Autodesk Inventor part; units mm, degrees
ref_plane "YZ Plane" through (0, 0, 0) normal (1, 0, 0) x (0, 1, 0)
ref_plane "XZ Plane" through (0, 0, 0) normal (0, 1, 0) x (-1, 0, 0)
ref_plane "XY Plane" through (0, 0, 0) normal (0, 0, 1) x (1, 0, 0)
sketch "Skizze1" plane through (0, 0, 0) normal (0, 0, 1) x (1, 0, 0)
  line L0 (0, 0) -> (50, 0)
  line L1 (50, 0) -> (50, 5)
  line L2 (36.2626, 10) -> (0, 10)
  line L3 (0, 10) -> (0, 0)
  line L4 (36.2626, 10) -> (50, 5)
  dimension "d0" = 10
  dimension "d1" = 50
  dimension "d2" = 5
  dimension "d5" = 20
extrude "Extrusion1" add sketch "Skizze1" along normal blind 2
sketch "Skizze2" plane through (0, 0, 2) normal (0, 0, 1) x (1, 0, 0)
  line L0 (0, 0) -> (0, 10)
  line L1 (0, 10) -> (36.2626, 10)
  line L2 (0, 5) -> (28.2614, 5)
  point P0 (4, 5)
  point P1 (12, 5)
  dimension "d8" = 4
  dimension "d9" = 8
hole "Bohrung1" at (4, 5, 2) at (12, 5, 2) direction (0, 0, -1) diameter 3.4 end through all
sketch "Skizze4" plane through (0, 0, 2) normal (0, 0, 1) x (1, 0, 0)
  circle A0 centre (4, 5) radius 1.7
  line L0 (50, 0) -> (0, 0)
  line L1 (0, 10) -> (36.2626, 10)
  line L2 (5.7, 7) -> (5.7, 3)
  line L3 (2.3, 3) -> (2.3, 7)
  arc A1 (5.7, 7) -> (2.3, 7) centre (4, 7) ccw
  arc A2 (2.3, 3) -> (5.7, 3) centre (4, 3) ccw
  dimension "d17" = 3
  dimension "d18" = 3
  dimension "d19" = 4
extrude "Extrusion2" cut sketch "Skizze4" against normal through all contours L2 A2 L3 A0 | A0 L3 A1 L2
pattern_linear "Rechteckige Anordnung1" count 2 spacing 8 along (1, 0, 0) of "Extrusion2"
properties part number "13_0204_068"
Design review of the part built by this model. Coordinates are the model's own, in mm. A direction names the side the tool comes from. Coordinates: 2 decimals unless noted, no trailing zeros. Write each loop counter-clockwise with the first axis right and the second up, starting at its lowest first coordinate (ties: lowest second). Pieces come first, ordered by that corner, then holes. Notation, with made-up numbers: (68, -13.5) - (113, -13.5) arc R8 ccw to (113, 1.5) - close; hole circle Ø6 at (-4, -22). An arc over 180 degrees is marked (long way). Use one line per item in the form item = value.
Q1. Insertion check: pin 1 Ø0.6 at (y, z) = (5.5, 1) entering from -X. The pin has a flat end and moves straight along its axis. Give the tip position at first contact, or say it passes through.
Taken from the geometry:
pin_1 = 0
Q2. Consider section C-C (z = 1.1). Write out the cut boundary in (x, y).
Taken from the geometry:
outline = (0, 0) - (50, 0) - (50, 5) - (36.26, 10) - (0, 10) - close; hole (2.3, 3) arc R1.7 ccw to (5.7, 3) - (5.7, 7) arc R1.7 ccw to (2.3, 7) - close; hole (10.3, 3) arc R1.7 ccw to (13.7, 3) - (13.7, 7) arc R1.7 ccw to (10.3, 7) - close
Q3. Consider section A-A (x = 12). Write out the cut boundary in (y, z), plus the area to 3 significant figures.
Taken from the geometry:
outline = (0, 0) - (1.3, 0) - (1.3, 2) - (0, 2) - close; (8.7, 0) - (10, 0) - (10, 2) - (8.7, 2) - close
area = 5.20 mm^2
Q4. For probe 1 along X at (y, z) = (4.5, 0.2); probe 2 along X at (y, z) = (1.5, 1.4); probe 3 along Y at (x, z) = (13.5, 1.8), list the stretches that pass through material, from the lowest coordinate up.
Taken from the geometry:
probe_1 = 0 to 2.3, 5.7 to 10.3, 13.7 to 50
probe_2 = 0 to 3.2, 4.8 to 11.2, 12.8 to 50
probe_3 = 0 to 2.2, 7.8 to 10
Q5. Consider section B-B (y = 4.25). Write out the cut boundary in (x, z), plus the area to 3 significant figures.
Taken from the geometry:
outline = (0, 0) - (2.3, 0) - (2.3, 2) - (0, 2) - close; (5.7, 0) - (10.3, 0) - (10.3, 2) - (5.7, 2) - close; (13.7, 0) - (50, 0) - (50, 2) - (13.7, 2) - close
area = 86.4 mm^2
Q6. The part is to be moulded in two halves that separate along Y. For faces 1 (the flat face through (25, 5, 0)), 2 (the cylindrical face through (12, 8.7, 1)), 3 (the flat face through (43.035, 7.535, 0.986)), say which applies: +Y half, -Y half, draft (parallel to the pull), parting line (faces both ways), or undercut.
Taken from the geometry:
face_1 = draft
face_2 = undercut
face_3 = +Y half
Q7. Consider section D-D (y = 2). Write out the cut boundary in (x, z), plus the area to 3 significant figures.
Taken from the geometry:
outline = (0, 0) - (2.63, 0) - (2.63, 2) - (0, 2) - close; (5.37, 0) - (10.63, 0) - (10.63, 2) - (5.37, 2) - close; (13.37, 0) - (50, 0) - (50, 2) - (13.37, 2) - close
area = 89.0 mm^2
Q8. Machinability: for faces 4 (the flat face through (0, 5, 1)), 5 (the flat face through (10.3, 5, 1)), which of the approach directions +Z, -Z, +X, -X, +Y, -Y give a long, thin tool a straight path to every point of the face, cutting with its end or side? Answer none if there is none.
Taken from the geometry:
face_4 = +Z, -Z, -X, +Y, -Y
face_5 = +Z, -Z
